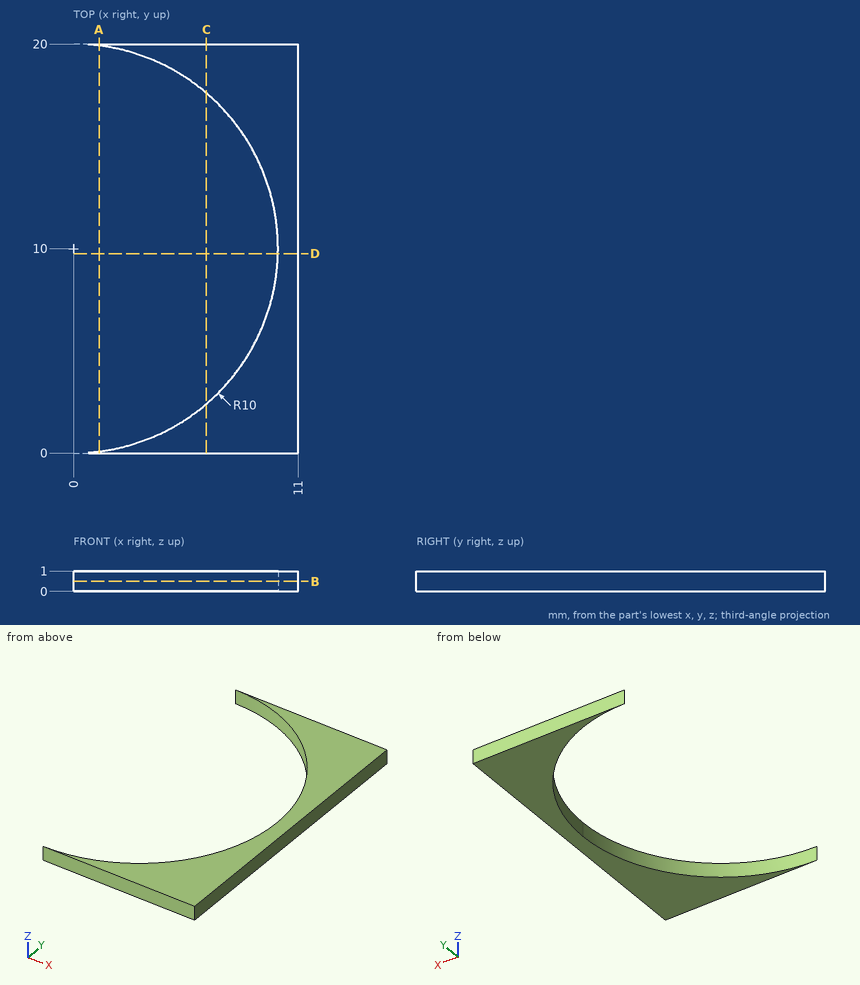
For this review, use the dimensioned drawing (mm, ordinates from the lowest corner) and the shaded views. Coordinates: 2 decimals unless noted, no trailing zeros. Loops run counter-clockwise (first coordinate to the right, second up) from the corner with the lowest first, then second, coordinate; pieces in that order, holes last. Notation, with made-up numbers: (82.25, 75.25) - (138.25, 75.25) arc R20 cw to (138.25, 85.25) - close; hole circle Ø2 at (25, -18). An arc over 180 degrees is marked (long way). Use one line per item in the form item = value. Start each with the question number.
1) Take a section at D-D (y = 9.75). State the section outline as (x, z) points.
2) Take a section at B-B (z = 0.5). State the section outline as (x, y) points.
3) Take a section at A-A (x = 1.25). State the section outline as (y, z) points.
4) Take a section at C-C (x = 6.5). State the section outline as (y, z) points.
5) To check wall thickness, follow probe 1 along Y at (x, z) = (2.5, 0.4); probe 2 along Y at (x, z) = (7.5, 0.8); probe 3 along X at (y, z) = (13.25, 0.45). State the ranges of each line that lie inside material, in increasing order. Write a range as from..to.
From the geometry:
q1.outline = (10, 0) - (11, 0) - (11, 1) - (10, 1) - close
q2.outline = (0, 0) - (11, 0) - (11, 20) - (0, 20) arc R10 cw to (10, 10) arc R10 cw to start
q3.outline = (0, 0) - (0.08, 0) - (0.08, 1) - (0, 1) - close; (19.92, 0) - (20, 0) - (20, 1) - (19.92, 1) - close
q4.outline = (0, 0) - (2.4, 0) - (2.4, 1) - (0, 1) - close; (17.6, 0) - (20, 0) - (20, 1) - (17.6, 1) - close
q5.probe_1 = 0..0.32, 19.68..20
q5.probe_2 = 0..3.39, 16.61..20
q5.probe_3 = 9.46..11
